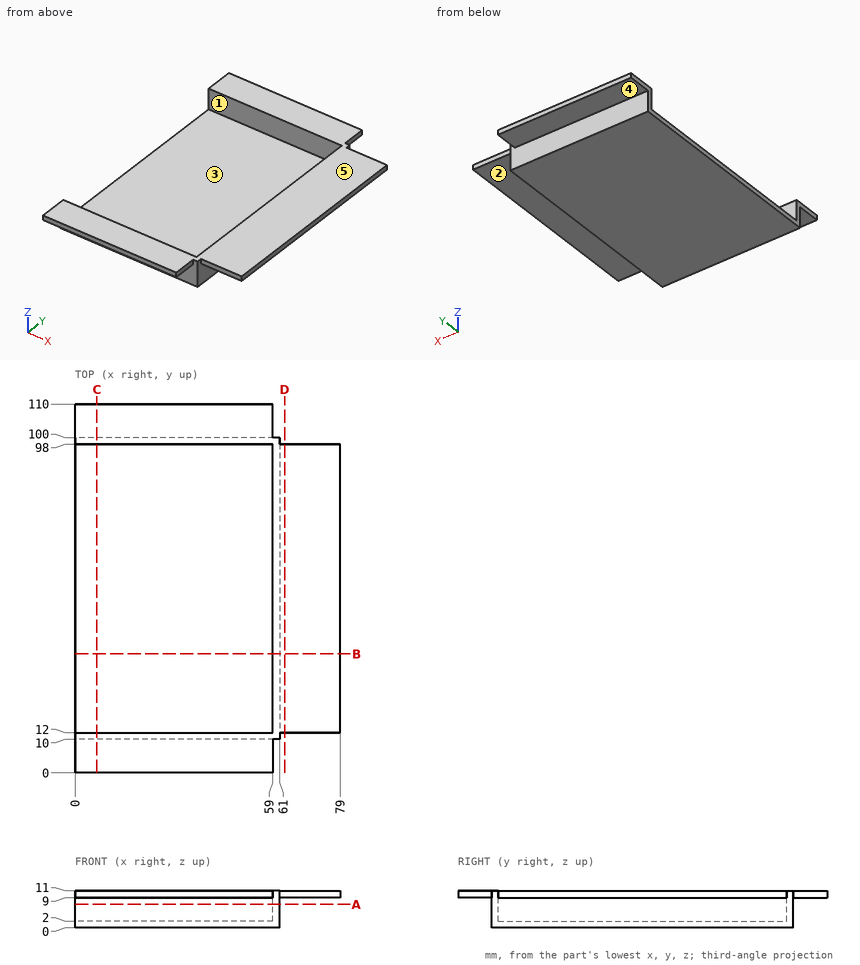
Input: dimensioned drawing with shaded views. Units: mm. Origin: part minimum x, y, z. A direction names the side the tool comes from. Give positions to 0.01 mm unless a question says otherwise; leave off trailing zeros. Loops run counter-clockwise (first coordinate to the right, second up) from the corner with the lowest first, then second, coordinate; pieces in that order, holes last. Notation, with made-up numbers: M 45,50 L 81,50 A23 ccw 81,59 Z; hole C -1,-22.75 d2. An arc over 180 degrees is marked long. Put each result on its own line as item: value.
1) Cut plane A-A, the plane z = 7. Return the cut outline in (x, y), plus the area to 3 significant figures.
Computed values:
outline: M 0,10 L 61,10 L 61,100 L 0,100 L 0,98 L 59,98 L 59,12 L 0,12 Z
area: 416 mm^2
2) Mould query, pull axis Y, two halves, no side actions, for the marked faces 1 and 2. Classes: released by +Y, released by -Y, zero draft, split by the parting line, or undercut.
Computed values:
face 1: undercut
face 2: zero draft
3) Cut plane D-D, the plane x = 62.5. Return the cut outline in (y, z).
Computed values:
outline: M 12,9 L 98,9 L 98,11 L 12,11 Z
4) Cut plane C-C, the plane x = 6.5. Return the cut outline in (y, z).
Computed values:
outline: M 0,9 L 10,9 L 10,0 L 100,0 L 100,9 L 110,9 L 110,11 L 98,11 L 98,2 L 12,2 L 12,11 L 0,11 Z
5) Cut plane B-B, the plane y = 35.5. Return the cut outline in (x, z), plus the area to 3 significant figures.
Computed values:
outline: M 0,0 L 61,0 L 61,9 L 79,9 L 79,11 L 59,11 L 59,2 L 0,2 Z
area: 176 mm^2
6) Reachability of the marked faces 3, 4 and 5 from +Z, -Z, +X, -X, +Y, -Y: full face, straight path, thin tool, end or side. Return the list, or none.
Computed values:
face 3: +Z, -X
face 4: -Z, +X, -X, +Y
face 5: +Z, +X, -X, +Y, -Y
7) First-contact query: P1, Ø5, axis at x = 13, z = 6, coming from the -Y side; P2, Ø1.5, axis at x = 24, y = 34.5, coming from the +Z side; P3, Ø11, axis at x = 40.5, y = 103, coming from the -Z side; P4, Ø1.5, axis at x = 14.5, z = 5, coming from the +Y side. Flat tips, straight axial feed; report the tip coordinate or a pass-through.
Computed values:
P1: stops at y = 10
P2: stops at z = 2
P3: stops at z = 0
P4: stops at y = 100
8) Material intervals for L1, parallel to Y at x = 43, z = 9.25; L2, parallel to Y at x = 42, z = 8.5; L3, parallel to X at y = 48.5, z = 1.25, sorted ascending. Write a range as from..to.
Computed values:
L1: y = 0..12, 98..110
L2: y = 10..12, 98..100
L3: x = 0..61
